The model under review builds one solid part; all positions refer to its coordinate system, in mm. A direction names the side the tool comes from. Coordinates: 2 decimals unless noted, no trailing zeros. Write each loop counter-clockwise with the first axis right and the second up, starting at its lowest first coordinate (ties: lowest second). Pieces come first, ordered by that corner, then holes. Notation, with made-up numbers: (-6, 61.25) - (15, 61.25) arc R24 ccw to (15, 86.25) - close; hole circle Ø8 at (87, 22.25). An arc over 180 degrees is marked (long way). Put each result on its own line as item: value.
Autodesk Inventor part; units mm, degrees
ref_plane "YZ Plane" through (0, 0, 0) normal (1, 0, 0) x (0, 1, 0)
ref_plane "XZ Plane" through (0, 0, 0) normal (0, 1, 0) x (-1, 0, 0)
ref_plane "XY Plane" through (0, 0, 0) normal (0, 0, 1) x (1, 0, 0)
sketch "Sketch1" plane through (0, 0, 0) normal (0, 0, 1) x (1, 0, 0)
  line L0 (-35.55, -33) -> (35.55, -33)
  line L1 (35.55, -33) -> (35.55, 33)
  line L2 (35.55, 33) -> (-35.55, 33)
  line L3 (-35.55, 33) -> (-35.55, -33)
  line L4 (-35.55, -33) -> (35.55, 33) construction
  line L5 (35.55, -33) -> (-35.55, 33) construction
  point P0 (0, 0)
  dimension "LENGTH" = 71.1
  dimension "WIDTH" = 66
extrude "Extrusion1" add sketch "Sketch1" along normal blind 10.16
sketch "Sketch2" plane through (0, 0, 0) normal (0, 0, 1) x (1, 0, 0)
  line L0 (46.55, -33) -> (-46.55, -33)
  line L1 (-46.55, -33) -> (-46.55, 33)
  line L2 (-46.55, 33) -> (46.55, 33)
  line L3 (46.55, 33) -> (46.55, -33)
  line L4 (46.55, -33) -> (-46.55, 33) construction
  line L5 (-46.55, -33) -> (46.55, 33) construction
  point P0 (0, 0)
  dimension "d4" = 93.1
  dimension "d5" = 66
extrude "Extrusion2" add sketch "Sketch2" along normal blind 5
sketch "Sketch3" plane through (0, 0, 5) normal (0, 0, 1) x (1, 0, 0)
  line L0 (-46.55, 33) -> (-46.55, -33)
  line L1 (46.55, -33) -> (46.55, 33)
  point P0 (0, 0)
  point P1 (-40.55, 0)
  point P2 (40.55, 0)
  dimension "d8" = 6
  dimension "d9" = 6
  dimension "d10" = 0
  dimension "d11" = 0
hole "Hole1" at (40.55, 0, 5) at (-40.55, 0, 5) direction (0, 0, -1) diameter 4.5 end through all counterbore diameter 8 counterbore depth 2
sketch "Sketch4" plane through (0, 0, 0) normal (0, 0, -1) x (-1, 0, 0)
  line L0 (-35.55, -33) -> (-35.55, 33)
  point P0 (0, 0)
  point P1 (-6.09, -25)
  point P2 (-6.09, 24.99)
  dimension "d19" = 25
  dimension "d20" = 49.99
  dimension "d21" = 29.46
  dimension "d22" = 29.46
hole "Hole2" at (6.09, -25, 0) at (6.09, 24.99, 0) direction (0, 0, 1) diameter 3.4 end through all counterbore diameter 6.5 counterbore depth 3
sketch "Sketch5" plane through (0, 0, 0) normal (0, 0, -1) x (-1, 0, 0)
  circle A0 centre (-6.09, 0) radius 15.875
  point P0 (0, 0)
  point P1 (-6.09, -15.875)
  point P2 (9.785, 0)
  point P3 (-6.09, 15.875)
  point P4 (-21.965, 0)
  dimension "d32" = 6.09
  dimension "d33" = 0
  dimension "d34" = 31.75
hole "Hole3" at (6.09, -15.875, 0) at (-9.785, 0, 0) at (6.09, 15.875, 0) at (21.965, 0, 0) direction (0, 0, 1) diameter 2.946 end through all counterbore diameter 5.558 counterbore depth 2.845
equation "\"d5\" = WIDTH"
properties part number "aom mount"
1. To check wall thickness, follow probe 1 along X at (y, z) = (0, 8.5); probe 2 along Y at (x, z) = (6.09, 6); probe 3 along X at (y, z) = (1, 4). State the ranges of each line that lie inside material, in increasing order.
Determined:
probe 1: x = -35.55 to -11.26, -8.31 to 20.49, 23.44 to 35.55
probe 2: y = -33 to -26.7, -23.3 to -17.35, -14.4 to 14.4, 17.35 to 23.29, 26.69 to 33
probe 3: x = -46.55 to -44.42, -36.68 to -10.87, -8.7 to 20.88, 23.05 to 36.68, 44.42 to 46.55
2. Machinability: for faces 1 (the flat face through (7.5, -23.6, 3)), 2 (the cylindrical face through (6.654, 17.236, 6.554)), 3 (the cylindrical face through (44.455, 0.867, 3.986)), which of the approach directions +Z, -Z, +X, -X, +Y, -Y give a long, thin tool a straight path to every point of the face, cutting with its end or side? Answer none if there is none.
Determined:
face 1: -Z
face 2: +Z, -Z
face 3: +Z
3. Consider section C-C on z = 7.5. State the section outline as (x, y) points (3 decimals), plus the area to 3 significant figures.
Determined:
outline: (-35.55, -33) - (35.55, -33) - (35.55, 33) - (-35.55, 33) - close; hole circle Ø2.946 at (-9.785, 0); hole circle Ø3.4 at (6.09, -25); hole circle Ø3.4 at (6.09, 24.99); hole circle Ø2.946 at (6.09, -15.875); hole circle Ø2.946 at (6.09, 15.875); hole circle Ø2.946 at (21.965, 0)
area: 4,650 mm^2
4. The part is to be moulded in two halves that separate along X. For faces 4 (the flat face through (1, 33, 5)), 5 (the flat face through (-35.55, 0, 8)), 6 (the flat face through (23.2, 1.2, 2.845)), say which applies: +X half, -X half, draft (parallel to the pull), parting line (faces both ways), or undercut.
Determined:
face 4: draft
face 5: -X half
face 6: undercut
5. Consider section A-A on y = 24.99. State the section outline as (x, z) points, plus the area to 3 significant figures.
Determined:
outline: (-46.55, 0) - (2.84, 0) - (2.84, 3) - (4.39, 3) - (4.39, 10.16) - (-35.55, 10.16) - (-35.55, 5) - (-46.55, 5) - close; (7.79, 3) - (9.34, 3) - (9.34, 0) - (46.55, 0) - (46.55, 5) - (35.55, 5) - (35.55, 10.16) - (7.79, 10.16) - close
area: 789 mm^2
6. Consider section B-B on x = 40.55. State the section outline as (y, z) points, plus the area to 4 significant figures.
Determined:
outline: (-33, 0) - (-2.25, 0) - (-2.25, 3) - (-4, 3) - (-4, 5) - (-33, 5) - close; (2.25, 0) - (33, 0) - (33, 5) - (4, 5) - (4, 3) - (2.25, 3) - close
area: 300.5 mm^2
7. Consider section D-D on y = 6.5. State the section outline as (x, z) points, plus the area to 3 significant figures.
Determined:
outline: (-46.55, 0) - (46.55, 0) - (46.55, 5) - (35.55, 5) - (35.55, 10.16) - (-35.55, 10.16) - (-35.55, 5) - (-46.55, 5) - close
area: 832 mm^2
8. For pin 1 Ø2.5 at (x, y) = (39.5, 0) entering from +Z; pin 2 Ø8 at (x, y) = (-8, -3) entering from -Z; pin 3 Ø2 at (y, z) = (24.5, 8) entering from -X; pin 4 Ø6 at (y, z) = (-9, 9) entering from +X, all flat-tipped, find the tip position at first contact; note any pin that passes through.
Determined:
pin 1: stops at z = 3
pin 2: stops at z = 0
pin 3: stops at x = -35.55
pin 4: stops at x = 35.55
